Read the model definition and answer for the solid it produces. Units are mm, in the model's axes. Face numbers are marked on the shaded views. A direction names the side the tool comes from. Coordinates: 2 decimals unless noted, no trailing zeros. Loops run counter-clockwise (first coordinate to the right, second up) from the corner with the lowest first, then second, coordinate; pieces in that order, holes last. Notation, with made-up numbers: (10.5, -5.75) -> (66.5, -5.75) arc R9 ccw to (66.5, 9.25) -> close; hole circle Ø5 at (84, 56.5). An arc over 180 degrees is marked (long way). Answer in a Markdown table with one row per item.
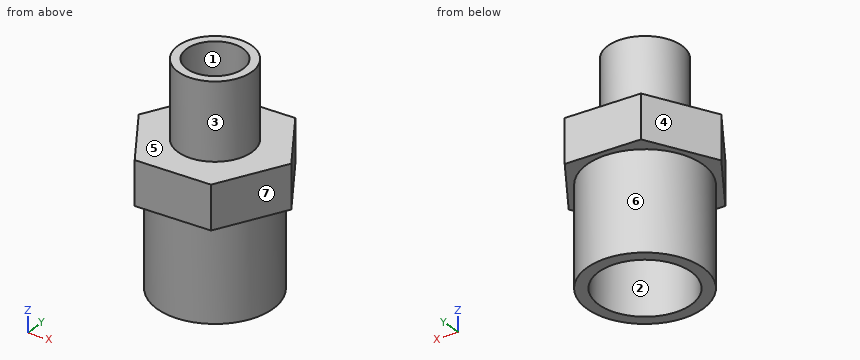
```python
from build123d import *

# Parameters (mm, degrees)
SKETCH1_R           = 8.5
SKETCH1_R_2         = 6.5
EXTRUDE_THIN1_DEPTH = 22.5
BOSS_EXTRUDE1_DEPTH = 5
SKETCH3_R           = 13.35
SKETCH3_R_2         = 10.65
EXTRUDE_THIN2_DEPTH = 22.5


with BuildPart() as part:
    # Sketch1 → Extrude-Thin1 (new body)
    with BuildSketch(Plane.XY):
        Circle(SKETCH1_R)
        Circle(SKETCH1_R_2, mode=Mode.SUBTRACT)
    extrude(amount=EXTRUDE_THIN1_DEPTH)

    # Sketch2 → Boss-Extrude1 (add, symmetric)
    with BuildSketch(Plane.XY):
        Polygon((17.021487729, 0.517918433), (8.062213344, 15), (-8.959274385, 14.482081567), (-17.021487729, -0.517918433), (-8.062213344, -15), (8.959274385, -14.482081567), align=None)
    extrude(amount=BOSS_EXTRUDE1_DEPTH, both=True)

    # Sketch3 → Extrude-Thin2 (add)
    with BuildSketch(Plane(origin=(0, 0, -5), x_dir=(-1, 0, 0), z_dir=(0, 0, -1))):
        Circle(SKETCH3_R)
        Circle(SKETCH3_R_2, mode=Mode.SUBTRACT)
    extrude(amount=EXTRUDE_THIN2_DEPTH)


solid = part.part
```
1. Given pin 1 Ø12 at (y, z) = (11, -21) entering from -X; pin 2 Ø15 at (x, y) = (-5.5, -2) entering from +Z; pin 3 Ø5 at (y, z) = (5.5, 16.5) entering from -X; pin 4 Ø8 at (y, z) = (10.5, 16) entering from -X, each flat-ended and moving along its own axis, determine where each tip first touches the part or whether it passes through.
A:
| item | result |
|---|---|
| pin 1 | stops at x = -12.38 |
| pin 2 | stops at z = 22.5 |
| pin 3 | stops at x = -7.95 |
| pin 4 | stops at x = -5.48 |
2. A cutting plane is placed at D-D on z = -1.5. Give the vertices of the cut face in (x, y), and give its area (3 significant figures).
A:
| item | result |
|---|---|
| outline | (-17.02, -0.52) -> (-8.06, -15) -> (8.96, -14.48) -> (17.02, 0.52) -> (8.06, 15) -> (-8.96, 14.48) -> close |
| area | 753 mm2 |
3. A cutting plane is placed at C-C on y = 7.5. Give the vertices of the cut face in (x, z), and give its area (3 significant figures).
A:
| item | result |
|---|---|
| outline | (-12.71, -5) -> (-11.04, -5) -> (-11.04, -27.5) -> (-7.56, -27.5) -> (-7.56, -5) -> (7.56, -5) -> (7.56, -27.5) -> (11.04, -27.5) -> (11.04, -5) -> (12.7, -5) -> (12.7, 5) -> (4, 5) -> (4, 22.5) -> (-4, 22.5) -> (-4, 5) -> (-12.71, 5) -> close |
| area | 551 mm2 |
4. A cutting plane is placed at A-A on z = 7.5. Give the vertices of the cut face in (x, y), and give its area (3 significant figures).
A:
| item | result |
|---|---|
| outline | circle Ø17 at (0, 0); hole circle Ø13 at (0, 0) |
| area | 94.2 mm2 |
5. Find the intervals of material crossed by probe 1 along Y at (x, z) = (0, 17.25); probe 2 along Z at (x, y) = (-6, -10), in increasing order.
A:
| item | result |
|---|---|
| probe 1 | y = -8.5 to -6.5, 6.5 to 8.5 |
| probe 2 | z = -27.5 to 5 |
6. A tool of negligible diameter and unlimited length cuts with its end or side. For the marked faces 5, 6 and 7, from which of +Z, -Z, +X, -X, +Y, -Y can it reach the whole face along a straight path? Write none if from no direction.
A:
| item | result |
|---|---|
| face 5 | +Z |
| face 6 | -Z |
| face 7 | +Z, -Z, +X, -Y |
7. The mould has two halves that part along Y. Classify the marked faces 1, 2, 3 and 4: pulls with the +Y half, pulls with the -Y half, needs draft (parallel to the pull), parting line crosses it, or undercut.
A:
| item | result |
|---|---|
| face 1 | undercut |
| face 2 | undercut |
| face 3 | parting line crosses it |
| face 4 | pulls with the +Y half |
8. A cutting plane is placed at B-B on x = -12.5. Give the vertices of the cut face in (y, z).
A:
| item | result |
|---|---|
| outline | (-7.83, -5) -> (-4.69, -5) -> (-4.69, -27.5) -> (4.69, -27.5) -> (4.69, -5) -> (7.89, -5) -> (7.89, 5) -> (-7.83, 5) -> close |
